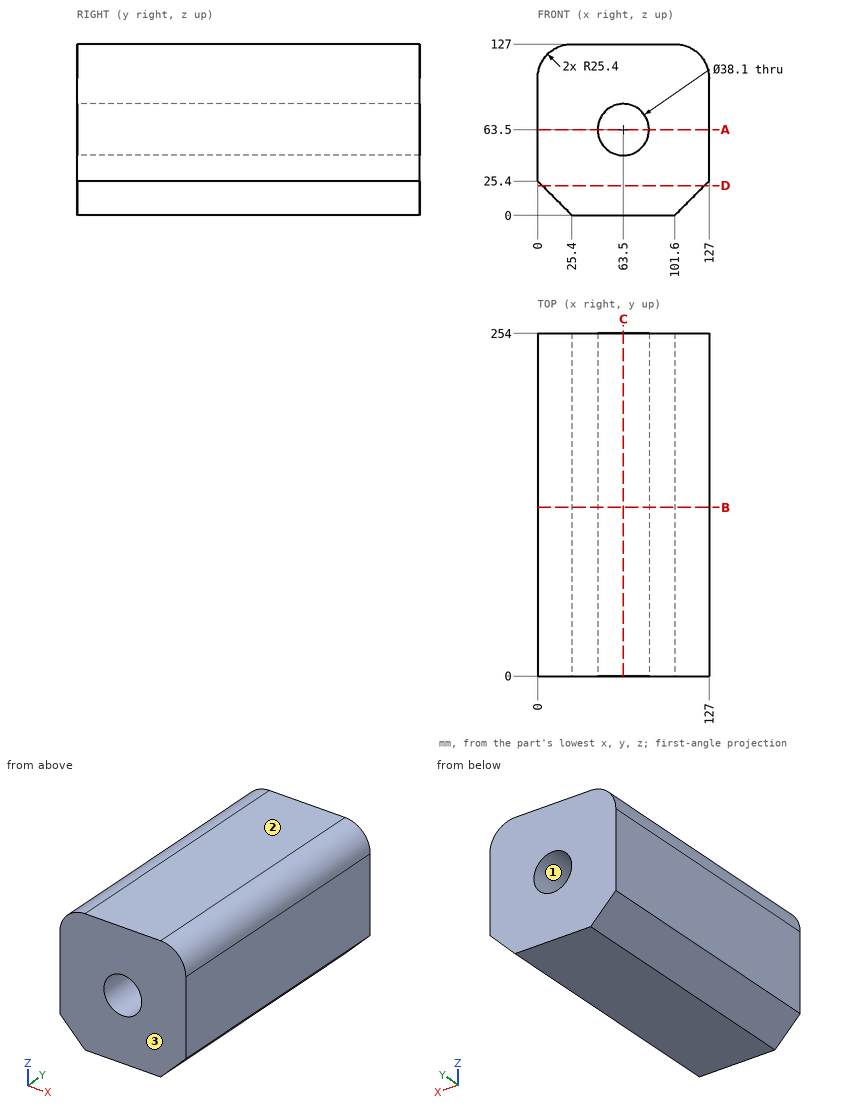
Geometry: see drawing. Coordinates: mm, zero at the bounding-box minimum. Coordinates: 2 decimals unless noted, no trailing zeros. Loops run counter-clockwise (first coordinate to the right, second up) from the corner with the lowest first, then second, coordinate; pieces in that order, holes last. Notation, with made-up numbers: M 85.5,64.5 L 128.5,64.5 A24 ccw 128.5,95.5 Z; hole C 11,-8 d8. An arc over 180 degrees is marked long. Answer in a Markdown table with one row per item.
1. Section B-B, the plane y = 125. Output: boundary loops of the cut face in (x, z).
Response:
| item | result |
|---|---|
| outline | M 0,25.4 L 25.4,0 L 101.6,0 L 127,25.4 L 127,101.6 A25.4 ccw 101.6,127 L 25.4,127 A25.4 ccw 0,101.6 Z; hole C 63.5,63.5 d38.1 |
2. Section D-D, the plane z = 22. Output: boundary loops of the cut face in (x, y).
Response:
| item | result |
|---|---|
| outline | M 3.4,0 L 123.6,0 L 123.6,254 L 3.4,254 Z |
3. First-contact query: pin 1 (3 mm diameter, centred on x = 20.5, y = 150, fed in from +Z); pin 2 (5 mm diameter, centred on x = 85, y = 225.5, fed in from -Z); pin 3 (1 mm diameter, centred on x = 113, y = 185, fed in from +Z); pin 4 (10 mm diameter, centred on x = 113.5, y = 171.5, fed in from -Z). Flat tips, straight axial feed; report the tip coordinate or a pass-through.
Response:
| item | result |
|---|---|
| pin 1 | stops at z = 126.77 |
| pin 2 | stops at z = 0 |
| pin 3 | stops at z = 124.54 |
| pin 4 | stops at z = 6.9 |
4. Section A-A, the plane z = 63.5. Output: boundary loops of the cut face in (x, y), then the cut area to 3 significant figures.
Response:
| item | result |
|---|---|
| outline | M 0,0 L 44.45,0 L 44.45,254 L 0,254 Z; M 82.55,0 L 127,0 L 127,254 L 82.55,254 Z |
| area | 22,600 mm2 |
5. Material intervals for line 1 (Z direction, x = 63, y = 86); line 2 (Z direction, x = 60.5, y = 201), sorted ascending.
Response:
| item | result |
|---|---|
| line 1 | z = 0 to 44.46, 82.54 to 127 |
| line 2 | z = 0 to 44.69, 82.31 to 127 |
6. Section C-C, the plane x = 63.5. Output: boundary loops of the cut face in (y, z).
Response:
| item | result |
|---|---|
| outline | M 0,0 L 254,0 L 254,44.45 L 0,44.45 Z; M 0,82.55 L 254,82.55 L 254,127 L 0,127 Z |
7. Draft query along Z for the marked faces 1, 2 and 3. Return one class per face: pulls with the +Z half, pulls with the -Z half, needs draft (parallel to the pull), parting line crosses it, or undercut.
Response:
| item | result |
|---|---|
| face 1 | undercut |
| face 2 | pulls with the +Z half |
| face 3 | needs draft |
